Verification items for the finished model (mm, model axes). Coordinates: 2 decimals unless noted, no trailing zeros. Order: outer loops, then holes, each group sorted by start corner. A loop starts at its lowest first (then second) coordinate and runs counter-clockwise, first axis right, second up. Notation, with made-up numbers: (14.5, 32) -> (59.5, 32) arc R19 ccw to (59.5, 52) -> close; hole circle Ø3 at (-39, 27). An arc over 180 degrees is marked (long way). Write each question's results on one line, items separated by ' | '. Start each with the question number.
(1) Cross-section at C-C on z = 65.5. Enter the section's corners in (x, y).
(2) Thickness scan on probe 1 along Y at (x, z) = (6, 30.5); probe 2 along Z at (x, y) = (4.75, -17.5); probe 3 along Y at (x, z) = (3.5, 87.5). Record the ranges inside material, lowest first. Write a range as [from, to].
(3) Draft check along Z on faces 1 (the flat face through (5, -78.5, 1)), 2 (the flat face through (5, 1, 96)), 3 (the cylindrical face through (4.684, 15.427, -31.822)). Enter one of: +Z half, -Z half, draft (parallel to the pull), parting line (faces both ways), or undercut.
(4) Cross-section at A-A on z = 87.5. Enter the section's corners in (x, y).
(5) Cross-section at B-B on y = 17.5. Enter the section's corners in (x, z).
(6) Go/stop test with a flat-tipped pin: pin 1 (5.5 mm diameter, centred on y = -17.5, z = 65.5, fed in from +X). Record where the tip stops, or that it passes through.
Autodesk Inventor part; units mm, degrees
ref_plane "YZ Plane" through (0, 0, 0) normal (1, 0, 0) x (0, 1, 0)
ref_plane "XZ Plane" through (0, 0, 0) normal (0, 1, 0) x (-1, 0, 0)
ref_plane "XY Plane" through (0, 0, 0) normal (0, 0, 1) x (1, 0, 0)
sketch "Skizze1" plane through (0, 0, 0) normal (1, 0, 0) x (0, 1, 0)
  line L0 (78.5, 96) -> (-78.5, 96)
  line L1 (-78.5, 96) -> (-78.5, -96)
  line L2 (-78.5, -96) -> (78.5, -96)
  line L3 (78.5, -96) -> (78.5, 96)
  point P0 (0, 0)
  dimension "d0" = 192
  dimension "d1" = 157
  dimension "d2" = 78.5
  dimension "d3" = 96
extrude "Extrusion1" add sketch "Skizze1" along normal blind 10
sketch "草图5" plane through (0, 0, 0) normal (-1, 0, 0) x (0, 0, 1)
  point P0 (0, 0)
sketch "草图6" plane through (10, 0, 0) normal (1, 0, 0) x (0, 0, -1)
  line L0 (-24, 25) -> (-72, 25)
  line L1 (-72, 25) -> (-72, -25)
  line L2 (-72, -25) -> (-24, -25)
  line L3 (-24, -25) -> (-24, 25)
  line L4 (-24, 25) -> (-72, -25) construction
  line L5 (-72, 25) -> (-24, -25) construction
  line L6 (-96, 78.5) -> (-96, -78.5)
  line L7 (-65.5, -17.5) -> (-30.5, -17.5)
  line L8 (-30.5, -17.5) -> (-30.5, 17.5)
  line L9 (-30.5, 17.5) -> (-65.5, 17.5)
  line L10 (-65.5, 17.5) -> (-65.5, -17.5)
  line L11 (-65.5, -17.5) -> (-30.5, 17.5) construction
  line L12 (-30.5, -17.5) -> (-65.5, 17.5) construction
  circle A0 centre (-65.5, -17.5) radius 2.5
  circle A1 centre (-30.5, -17.5) radius 2.5
  circle A2 centre (-30.5, 17.5) radius 2.5
  circle A3 centre (-65.5, 17.5) radius 2.5
  line L13 (24, 25) -> (72, 25)
  line L14 (72, 25) -> (72, -25)
  line L15 (72, -25) -> (24, -25)
  line L16 (24, -25) -> (24, 25)
  line L17 (24, 25) -> (72, -25) construction
  line L18 (72, 25) -> (24, -25) construction
  line L19 (65.5, -17.5) -> (30.5, -17.5)
  line L20 (30.5, -17.5) -> (30.5, 17.5)
  line L21 (30.5, 17.5) -> (65.5, 17.5)
  line L22 (65.5, 17.5) -> (65.5, -17.5)
  line L23 (65.5, -17.5) -> (30.5, 17.5) construction
  line L24 (30.5, -17.5) -> (65.5, 17.5) construction
  circle A4 centre (65.5, -17.5) radius 2.5
  circle A5 centre (30.5, -17.5) radius 2.5
  circle A6 centre (30.5, 17.5) radius 2.5
  circle A7 centre (65.5, 17.5) radius 2.5
  point P0 (0, 0)
  point P1 (-48, 0)
  point P2 (-48, 0)
  point P3 (48, 0)
  point P4 (48, 0)
  dimension "d31" = 50
  dimension "d32" = 48
  dimension "d33" = 24
  dimension "d34" = 35
  dimension "d35" = 35
  dimension "d36" = 5
  dimension "d39" = 360
  dimension "d48" = 5
  dimension "d49" = 5
  dimension "d50" = 5
  dimension "d51" = 5
hole "孔1" at (10, -17.5, 65.5) at (10, 17.5, 65.5) at (10, -17.5, 30.5) at (10, -17.5, -30.5) at (10, 17.5, -30.5) at (10, 17.5, -65.5) at (10, -17.5, -65.5) at (10, 17.5, 65.5) at (10, 17.5, 30.5) direction (-1, 0, 0) diameter 4.917 end through all
chamfer "倒角1" distance 0.5 angle 45 8 edges at (10, -17.5, -63.0415) (10, -17.5, -28.0415) (10, 17.5, -63.0415) (10, 17.5, -28.0415) (10, -17.5, 32.9585) (10, -17.5, 67.9585) (10, 17.5, 32.9585) (10, 17.5, 67.9585)
sketch "草图10" plane through (10, 0, 0) normal (1, 0, 0) x (0, 0, -1)
  line L0 (-169, 0) -> (145, 0)
  line L1 (0, 114) -> (0, -130)
  line L2 (-96, 78.5) -> (-96, -78.5)
  line L3 (-87.5, 62.5) -> (87.5, 62.5)
  line L4 (87.5, 62.5) -> (87.5, -62.5)
  line L5 (87.5, -62.5) -> (-87.5, -62.5)
  line L6 (-87.5, -62.5) -> (-87.5, 62.5)
  line L7 (-87.5, 62.5) -> (87.5, -62.5) construction
  line L8 (87.5, 62.5) -> (-87.5, -62.5) construction
  circle A0 centre (-87.5, 62.5) radius 3.25
  circle A1 centre (-87.5, -62.5) radius 3.25
  circle A2 centre (87.5, 62.5) radius 3.25
  circle A3 centre (87.5, -62.5) radius 3.25
  point P0 (0, 0)
  dimension "d74" = 96
  dimension "d75" = 175
  dimension "d76" = 125
  dimension "d77" = 6.5
extrude "拉伸5" cut sketch "草图10" against normal blind 10 contours A1 L5 L6 | L6 L5 A1 | A0 L3 L6 | L6 L3 A0 | A2 L3 L4 | L4 L3 A2 | A3 L5 L4 | L4 L5 A3
thread "螺纹6"
thread "螺纹7"
thread "螺纹8"
thread "螺纹9"
chamfer "倒角4" distance 0.2 angle 45 4 edges at (10, -62.5, 90.75) (10, -62.5, -84.25) (10, 62.5, -84.25) (10, 62.5, 90.75)
properties part number "Adapterplatte1Gong_2025-03-28v00r00grm"
Results are:
1) outline: (0, -78.5) -> (10, -78.5) -> (10, -20.46) -> (9.5, -19.96) -> (0, -19.96) -> close; (0, -15.04) -> (9.5, -15.04) -> (10, -14.54) -> (10, 14.54) -> (9.5, 15.04) -> (0, 15.04) -> close; (0, 19.96) -> (9.5, 19.96) -> (10, 20.46) -> (10, 78.5) -> (0, 78.5) -> close
2) probe 1: y = [-78.5, -19.96], [-15.04, 15.04], [19.96, 78.5] | probe 2: z = [-96, -67.96], [-63.04, -32.96], [-28.04, 28.04], [32.96, 63.04], [67.96, 96] | probe 3: y = [-78.5, -65.75], [-59.25, 59.25], [65.75, 78.5]
3) face 1: draft | face 2: +Z half | face 3: undercut
4) outline: (0, -78.5) -> (10, -78.5) -> (10, -65.95) -> (9.8, -65.75) -> (0, -65.75) -> close; (0, -59.25) -> (9.8, -59.25) -> (10, -59.05) -> (10, 59.05) -> (9.8, 59.25) -> (0, 59.25) -> close; (0, 65.75) -> (9.8, 65.75) -> (10, 65.95) -> (10, 78.5) -> (0, 78.5) -> close
5) outline: (0, -96) -> (10, -96) -> (10, -68.46) -> (9.5, -67.96) -> (0, -67.96) -> close; (0, -63.04) -> (9.5, -63.04) -> (10, -62.54) -> (10, -33.46) -> (9.5, -32.96) -> (0, -32.96) -> close; (0, -28.04) -> (9.5, -28.04) -> (10, -27.54) -> (10, 27.54) -> (9.5, 28.04) -> (0, 28.04) -> close; (0, 32.96) -> (9.5, 32.96) -> (10, 33.46) -> (10, 62.54) -> (9.5, 63.04) -> (0, 63.04) -> close; (0, 67.96) -> (9.5, 67.96) -> (10, 68.46) -> (10, 96) -> (0, 96) -> close
6) pin 1: stops at x = 9.79
